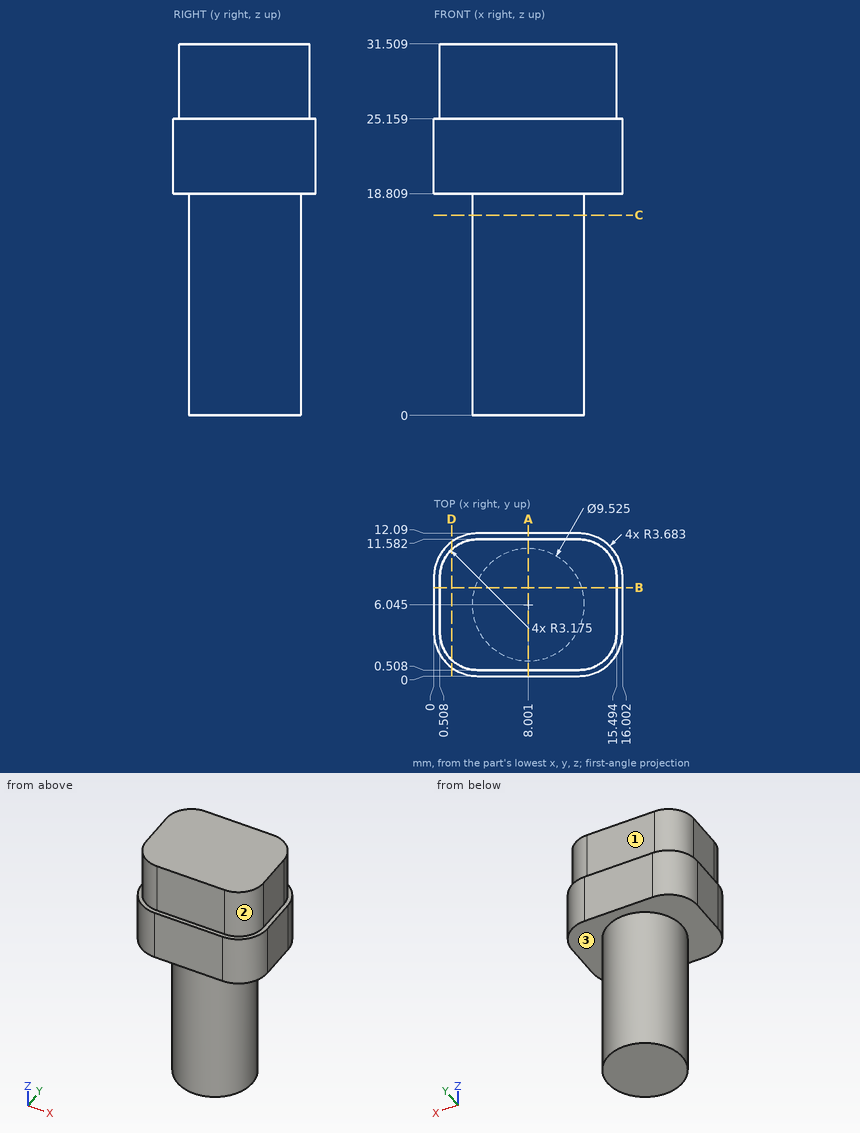
For this review, use the dimensioned drawing (mm, ordinates from the lowest corner) and the shaded views. A direction names the side the tool comes from. Give positions to 0.01 mm unless a question says otherwise; leave off trailing zeros. Loops run counter-clockwise (first coordinate to the right, second up) from the corner with the lowest first, then second, coordinate; pieces in that order, holes last.
Item 1: For line 1 along Z through (x, y) = (13.75, 9.75); line 2 along Z through (x, y) = (14, 11.25); line 3 along X through (y, z) = (6, 27), list the stretches that pass through material, from the lowest coordinate up.
Item 2: Insertion check: pin 1 (4 mm diameter, centred on y = 5.5, z = 29.5, fed in from +X); pin 2 (5 mm diameter, centred on y = 10.5, z = 15.5, fed in from -X); pin 3 (1.4 mm diameter, centred on y = 5.5, z = 27.5, fed in from -X). Each pin has a flat end and moves straight along its axis. Give the tip position at first contact, or say it passes through.
Item 3: Take a section at B-B, the plane y = 7.5. State the section outline as (x, z) points, and give its area (3 significant figures).
Item 4: Take a section at C-C, the plane z = 17. State the section outline as (x, y) points (1 decimal).
Item 5: Take a section at D-D, the plane x = 1.5. State the section outline as (y, z) points.
Item 6: Tool access review of the marked faces 1, 2 and 3: name each direction out of +Z, -Z, +X, -X, +Y, -Y from which nothing blocks a thin tool from reaching the whole face with its end or side.
Item 7: Take a section at A-A, the plane x = 8. State the section outline as (y, z) points.
Calculated:
1. line 1: z = 18.81 to 31.51
1. line 2: z = 18.81 to 25.16
1. line 3: x = 0.51 to 15.49
2. pin 1: stops at x = 15.49
2. pin 2: stops at x = 3.66
2. pin 3: stops at x = 0.51
3. outline: (0, 18.81) - (3.47, 18.81) - (3.47, 0) - (12.54, 0) - (12.54, 18.81) - (16, 18.81) - (16, 25.16) - (15.49, 25.16) - (15.49, 31.51) - (0.51, 31.51) - (0.51, 25.16) - (0, 25.16) - close
3. area: 367 mm2
4. outline: circle Ø9.5 at (8, 6)
5. outline: (0.72, 18.81) - (11.37, 18.81) - (11.37, 25.16) - (10.71, 25.16) - (10.71, 31.51) - (1.38, 31.51) - (1.38, 25.16) - (0.72, 25.16) - close
6. face 1: +Z, +X, -X, +Y
6. face 2: +Z, +X, -Y
6. face 3: -Z
7. outline: (0, 18.81) - (1.28, 18.81) - (1.28, 0) - (10.81, 0) - (10.81, 18.81) - (12.09, 18.81) - (12.09, 25.16) - (11.58, 25.16) - (11.58, 31.51) - (0.51, 31.51) - (0.51, 25.16) - (0, 25.16) - close
